Job drawing, mm, ordinate dimensions from the low corner. One solid piece. Give positions to 0.01 mm unless a question says otherwise; leave off trailing zeros. Order: outer loops, then holes, each group sorted by start corner. A loop starts at its lowest first (then second) coordinate and runs counter-clockwise, first axis right, second up. Notation, with made-up numbers: M -21,70 L -4,70 A24 cw -4,96 Z; hole C 35.5,25 d10. An arc over 180 degrees is marked long. One line per question, with ' | ' between items.
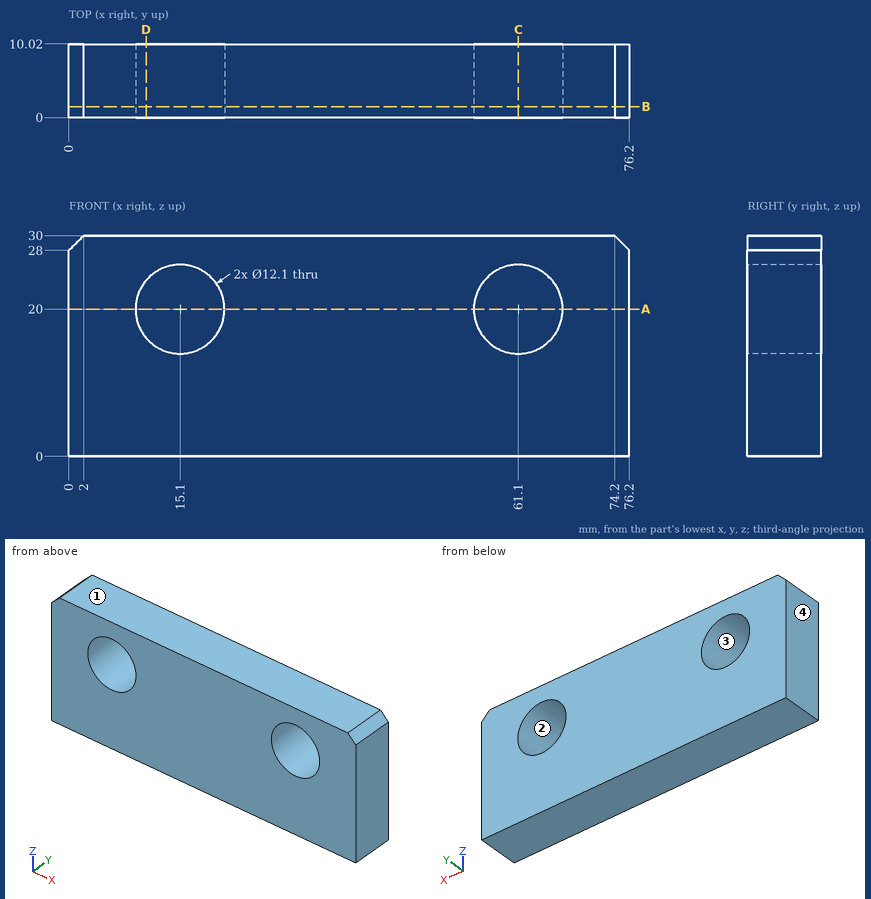
1. Mould opens along Z. For the marked faces 1, 2, 3 and 4 say: released by +Z, released by -Z, zero draft, split by the parting line, or undercut.
Worked out:
face 1: released by +Z | face 2: undercut | face 3: undercut | face 4: zero draft
2. Slice it at A-A on z = 20. Give the cut face in (x, y), then the cut area to 3 significant figures.
Worked out:
outline: M 0,0 L 9.05,0 L 9.05,10.02 L 0,10.02 Z; M 21.15,0 L 55.05,0 L 55.05,10.02 L 21.15,10.02 Z; M 67.15,0 L 76.2,0 L 76.2,10.02 L 67.15,10.02 Z | area: 521 mm2
3. Slice it at D-D on x = 10.5. Give the cut face in (y, z).
Worked out:
outline: M 0,0 L 10.02,0 L 10.02,16.07 L 0,16.07 Z; M 0,23.93 L 10.02,23.93 L 10.02,30 L 0,30 Z
4. Slice it at C-C on x = 61.1. Give the cut face in (y, z).
Worked out:
outline: M 0,0 L 10.02,0 L 10.02,13.95 L 0,13.95 Z; M 0,26.05 L 10.02,26.05 L 10.02,30 L 0,30 Z
5. Slice it at B-B on y = 1.5. Give the cut face in (x, z).
Worked out:
outline: M 0,0 L 76.2,0 L 76.2,28 L 74.2,30 L 2,30 L 0,28 Z; hole C 15.1,20 d12.1; hole C 61.1,20 d12.1
6. Probe L1, parallel to X at y = 2.25, z = 20; L2, parallel to Z at x = 61.1, y = 4.5; L3, parallel to X at y = 2.25, z = 16.5. List the from-to ranges inside material, lowest first. Write a range as from..to.
Worked out:
L1: x = 0..9.05, 21.15..55.05, 67.15..76.2 | L2: z = 0..13.95, 26.05..30 | L3: x = 0..10.17, 20.03..56.17, 66.03..76.2
7. Drop a flat-ended pin along its axis: pin 1 (7.5 mm diameter, centred on x = 15.1, z = 20, fed in from +Y). Give the stop position or say it passes through.
Worked out:
pin 1: passes through
